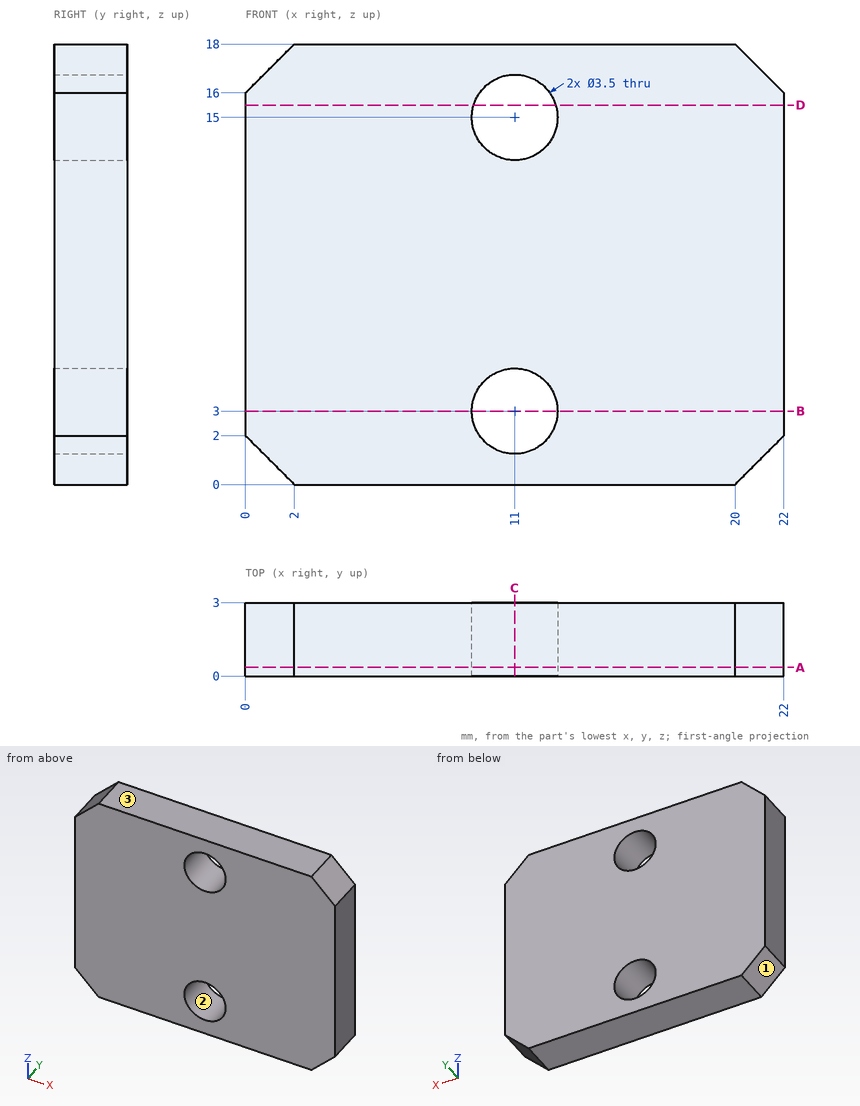
Could you check a few things on this drawing? It's one solid part, dimensions in mm from its lowest x, y, z. Give positions to 0.01 mm unless a question says otherwise; leave off trailing zeros. Order: outer loops, then holes, each group sorted by start corner. A loop starts at its lowest first (then second) coordinate and runs counter-clockwise, first axis right, second up. Notation, with made-up numbers: (1, 9) - (14, 9) arc R25 ccw to (14, 27) - close; hole circle Ø11 at (64, -16.75). An arc over 180 degrees is marked (long way). One line per question, with ' | ' between items. Start each with the question number.
Item 1: I want a section at D-D on z = 15.5. Write out the boundary of the cut face in (x, y), then the cut area to 3 significant figures.
Item 2: I need wall thicknesses on probe 1 along Z at (x, y) = (11, 0.95); probe 2 along Z at (x, y) = (12, 2.3); probe 3 along X at (y, z) = (1.25, 15). Which ranges of each line are inside material? Lowest first, please. Write a range as [from, to].
Item 3: I want a section at A-A on y = 0.35. Write out the boundary of the cut face in (x, z).
Item 4: I want a section at C-C on x = 11. Write out the boundary of the cut face in (y, z).
Item 5: Thinking about a two-plate mould opening in Z: for the marked faces 1, 2 and 3, which applies, pulls with the +Z half, pulls with the -Z half, needs draft (parallel to the pull), parting line crosses it, or undercut?
Item 6: I want a section at B-B on z = 3. Write out the boundary of the cut face in (x, y).
Verdict:
1) outline: (0, 0) - (9.32, 0) - (9.32, 3) - (0, 3) - close; (12.68, 0) - (22, 0) - (22, 3) - (12.68, 3) - close | area: 55.9 mm^2
2) probe 1: [0, 1.25], [4.75, 13.25], [16.75, 18] | probe 2: [0, 1.56], [4.44, 13.56], [16.44, 18] | probe 3: [0, 9.25], [12.75, 22]
3) outline: (0, 2) - (2, 0) - (20, 0) - (22, 2) - (22, 16) - (20, 18) - (2, 18) - (0, 16) - close; hole circle Ø3.5 at (11, 3); hole circle Ø3.5 at (11, 15)
4) outline: (0, 0) - (3, 0) - (3, 1.25) - (0, 1.25) - close; (0, 4.75) - (3, 4.75) - (3, 13.25) - (0, 13.25) - close; (0, 16.75) - (3, 16.75) - (3, 18) - (0, 18) - close
5) face 1: pulls with the -Z half | face 2: undercut | face 3: pulls with the +Z half
6) outline: (0, 0) - (9.25, 0) - (9.25, 3) - (0, 3) - close; (12.75, 0) - (22, 0) - (22, 3) - (12.75, 3) - close
